Work out the finished part from the listing and answer in its coordinate system (mm). Round coordinates to 2 decimals unless told otherwise and drop trailing zeros. Loops run counter-clockwise (first coordinate to the right, second up) from the corner with the lowest first, then second, coordinate; pieces in that order, holes last.
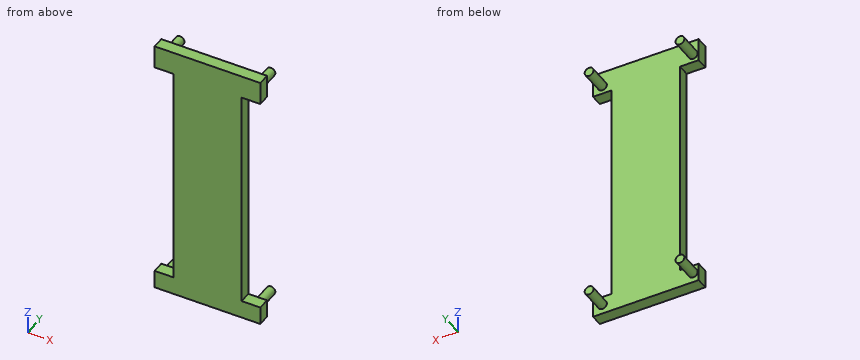
```python
from build123d import *

# Parameters (mm, degrees)
SKETCH1_W           = 17.9
SKETCH1_H           = 45
BOSS_EXTRUDE1_DEPTH = 2
SKETCH2_R           = 0.75
BOSS_EXTRUDE2_DEPTH = 4
SKETCH4_W           = 3.16
SKETCH4_H           = 38
CUT_EXTRUDE1_DEPTH  = 3.5


with BuildPart() as part:
    # Sketch1 → Boss-Extrude1 (new body)
    with BuildSketch(Plane(origin=(0, 0, 0), x_dir=(1, 0, 0), z_dir=(0, 1, 0))):
        with Locations((8.95, 22.5)):
            Rectangle(SKETCH1_W, SKETCH1_H)
    extrude(amount=BOSS_EXTRUDE1_DEPTH)

    # Sketch2 → Boss-Extrude2 (add)
    with BuildSketch(Plane(origin=(0, 2, 0), x_dir=(1, 0, 0), z_dir=(0, 1, 0))):
        with Locations((0.913071853, 43.396593807)):
            Circle(SKETCH2_R)
        with Locations((16.300481816, 43.396593807)):
            Circle(SKETCH2_R)
        with Locations((16.300481816, 2.58)):
            Circle(SKETCH2_R)
        with Locations((0.913071853, 2.58)):
            Circle(SKETCH2_R)
    extrude(amount=BOSS_EXTRUDE2_DEPTH)

    # Sketch4 → Cut-Extrude1 (cut)
    with BuildSketch(Plane(origin=(0, 2, 0), x_dir=(1, 0, 0), z_dir=(0, 1, 0))):
        with Locations((1.58, 22.925686587)):
            Rectangle(SKETCH4_W, SKETCH4_H)
        with Locations((16.32, 22.925686587)):
            Rectangle(SKETCH4_W, SKETCH4_H)
    extrude(amount=-CUT_EXTRUDE1_DEPTH, mode=Mode.SUBTRACT)


solid = part.part
```
1. Given pin 1 (5 mm diameter, centred on x = 11.5, z = -36.5, fed in from +Y); pin 2 (1.6 mm diameter, centred on y = 1, z = -21.5, fed in from +X); pin 3 (1 mm diameter, centred on y = 1, z = -29, fed in from -X), each flat-ended and moving along its own axis, determine where each tip first touches the part or whether it passes through.
Answer key:
pin 1: stops at y = 2
pin 2: stops at x = 14.74
pin 3: stops at x = 3.16
2. Find section A-A (z = -2.58). Write down the section's boundary in (x, y), then the cut area to 3 significant figures.
Answer key:
outline: (0, 0) - (17.9, 0) - (17.9, 2) - (17.05, 2) - (17.05, 6) - (15.55, 6) - (15.55, 2) - (1.66, 2) - (1.66, 6) - (0.16, 6) - (0.16, 2) - (0, 2) - close
area: 47.8 mm2
3. Find section B-B (x = 12.25). Write down the section's boundary in (y, z), then the cut area to 3 significant figures.
Answer key:
outline: (0, -45) - (2, -45) - (2, 0) - (0, 0) - close
area: 90.0 mm2
4. Find section C-C (y = 3.8). Write down the section's boundary in (x, z), then the cut area to 3 significant figures.
Answer key:
outline: circle Ø1.5 at (0.91, -43.4); circle Ø1.5 at (0.91, -2.58); circle Ø1.5 at (16.3, -43.4); circle Ø1.5 at (16.3, -2.58)
area: 7.07 mm2
5. Consider probe 1 along Z at (x, y) = (16, 1.7); probe 2 along Z at (x, y) = (1, 2.6); probe 3 along X at (y, z) = (1.1, -27). Determine where each line is inside the solid, lowest interval first.
Answer key:
probe 1: z = -45 to -41.93, -3.93 to 0
probe 2: z = -44.14 to -42.65, -3.32 to -1.84
probe 3: x = 3.16 to 14.74
6. Find section D-D (z = -11). Write down the section's boundary in (x, y).
Answer key:
outline: (3.16, 0) - (14.74, 0) - (14.74, 2) - (3.16, 2) - close
